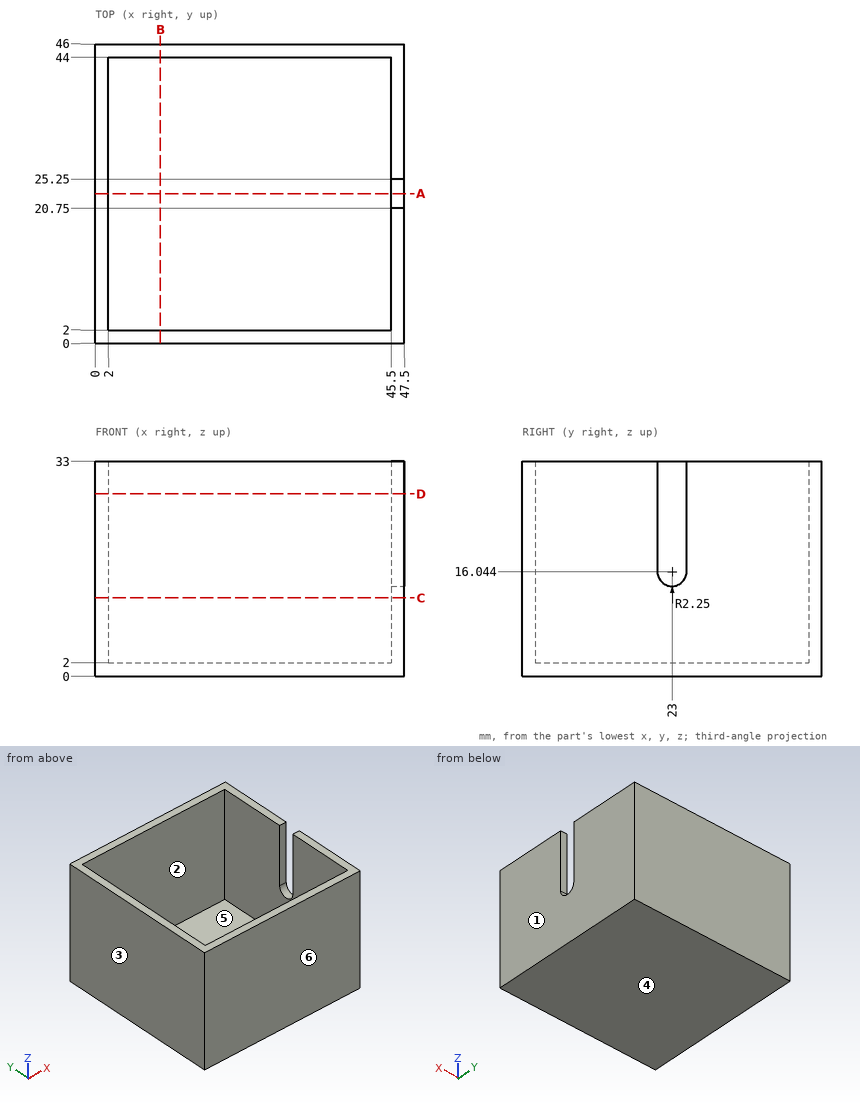
Job drawing, mm, ordinate dimensions from the low corner. One solid piece. A direction names the side the tool comes from. Coordinates: 2 decimals unless noted, no trailing zeros. Loops run counter-clockwise (first coordinate to the right, second up) from the corner with the lowest first, then second, coordinate; pieces in that order, holes last. Notation, with made-up numbers: (58, 76.25) - (75, 76.25) arc R19 ccw to (75, 107.25) - close; hole circle Ø11 at (-38, -23.5). An arc over 180 degrees is marked (long way). Answer as a JSON object with one key per item and string values. Group by question number.
(1) Cut at B-B (x = 10). Give the cut face in (y, z).
(2) Flat gauge pin, fed straight in: pin 1 (3 mm diameter, centred on x = 27, y = 11, fed in from +Z). Where does the tip first touch, or does it go through?
(3) Cut at C-C (z = 12). Give the cut face in (x, y).
(4) Tool access for the marked faces 5 and 6: list every direction of +Z, -Z, +X, -X, +Y, -Y with a clear straight run to the whole face (end or side of a thin tool).
(5) Cut at D-D (z = 28). Give the cut face in (x, y).
(6) Cut at A-A (y = 23). Give the cut face in (x, z).
(7) Probe line 1 along Y through (x, z) = (41, 28.5); line 2 along X through (y, z) = (34, 13); line 3 along Z through (x, y) = (41, 10.5). List the from-to ranges inside material, lowest first.
(8) Two-plate mould, pull along X, no slides. Class the marked faces 1, 2, 3 and 4: released by +X, released by -X, zero draft, split by the parting line, or undercut.
Geometry says:
{
 "1": {"outline": "(0, 0) - (46, 0) - (46, 33) - (44, 33) - (44, 2) - (2, 2) - (2, 33) - (0, 33) - close"},
 "2": {"pin 1": "stops at z = 2"},
 "3": {"outline": "(0, 0) - (47.5, 0) - (47.5, 46) - (0, 46) - close; hole (2, 2) - (45.5, 2) - (45.5, 44) - (2, 44) - close"},
 "4": {"face 5": "+Z", "face 6": "+Z, -Z, +X, -X, -Y"},
 "5": {"outline": "(0, 0) - (47.5, 0) - (47.5, 20.75) - (45.5, 20.75) - (45.5, 2) - (2, 2) - (2, 44) - (45.5, 44) - (45.5, 25.25) - (47.5, 25.25) - (47.5, 46) - (0, 46) - close"},
 "6": {"outline": "(0, 0) - (47.5, 0) - (47.5, 13.79) - (45.5, 13.79) - (45.5, 2) - (2, 2) - (2, 33) - (0, 33) - close"},
 "7": {"line 1": "y = 0 to 2, 44 to 46", "line 2": "x = 0 to 2, 45.5 to 47.5", "line 3": "z = 0 to 2"},
 "8": {"face 1": "released by +X", "face 2": "undercut", "face 3": "released by -X", "face 4": "zero draft"}
}
